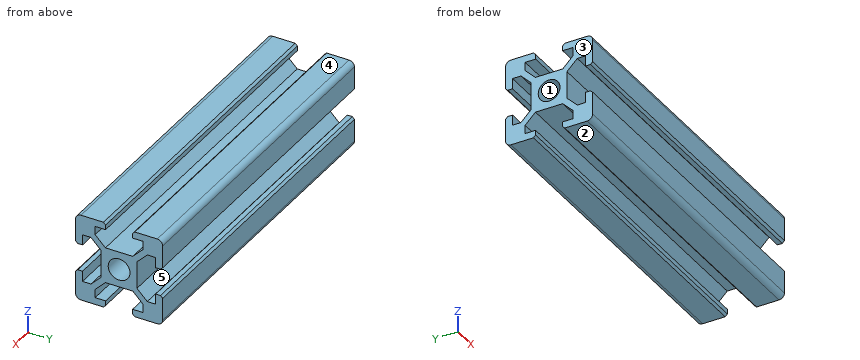
Autodesk Inventor part; units mm, degrees
ref_plane "YZ Plane" through (0, 0, 0) normal (1, 0, 0) x (0, 1, 0)
ref_plane "XZ Plane" through (0, 0, 0) normal (0, 1, 0) x (-1, 0, 0)
ref_plane "XY Plane" through (0, 0, 0) normal (0, 0, 1) x (1, 0, 0)
sketch "Sketch1" plane through (0, 0, 0) normal (1, 0, 0) x (0, 1, 0)
  circle A0 centre (0, 0) radius 2.5
  line L0 (0, 0) -> (10, 0)
  line L1 (10, -10) -> (10, -3.6)
  line L2 (10, -3.6) -> (9.5, -3.1)
  line L3 (9.5, -3.1) -> (8.4, -3.1)
  line L4 (8.4, -3.1) -> (8.4, -5.5)
  line L5 (-3.134, 4.1) -> (3.134, 4.1)
  line L6 (4.1, 3.134) -> (4.1, -3.134)
  line L7 (3.134, -4.1) -> (-3.134, -4.1)
  line L8 (-4.1, -3.134) -> (-4.1, 3.134)
  line L9 (-4.1, 4.1) -> (4.1, -4.1) construction
  line L10 (4.1, 4.1) -> (-4.1, -4.1) construction
  line L11 (4.1, -3.134) -> (6.466, -5.5)
  line L12 (8.4, -5.5) -> (6.466, -5.5)
  line L13 (10, -10) -> (3.6, -10)
  line L14 (3.6, -10) -> (3.1, -9.5)
  line L15 (3.1, -9.5) -> (3.1, -8.4)
  line L16 (3.1, -8.4) -> (5.5, -8.4)
  line L17 (3.134, -4.1) -> (5.5, -6.466)
  line L18 (5.5, -8.4) -> (5.5, -6.466)
  line L19 (10, 10) -> (10, 3.6)
  line L20 (10, 3.6) -> (9.5, 3.1)
  line L21 (9.5, 3.1) -> (8.4, 3.1)
  line L22 (8.4, 3.1) -> (8.4, 5.5)
  line L23 (4.1, 3.134) -> (6.466, 5.5)
  line L24 (8.4, 5.5) -> (6.466, 5.5)
  line L25 (5.5, 8.4) -> (5.5, 6.466)
  line L26 (3.134, 4.1) -> (5.5, 6.466)
  line L27 (3.1, 8.4) -> (5.5, 8.4)
  line L28 (3.1, 9.5) -> (3.1, 8.4)
  line L29 (3.6, 10) -> (3.1, 9.5)
  line L30 (10, 10) -> (3.6, 10)
  line L31 (0, 0) -> (0, -5.5)
  line L32 (-10, -10) -> (-10, -3.6)
  line L33 (-10, -3.6) -> (-9.5, -3.1)
  line L34 (-9.5, -3.1) -> (-8.4, -3.1)
  line L35 (-8.4, -3.1) -> (-8.4, -5.5)
  line L36 (-4.1, -3.134) -> (-6.466, -5.5)
  line L37 (-8.4, -5.5) -> (-6.466, -5.5)
  line L38 (-5.5, -8.4) -> (-5.5, -6.466)
  line L39 (-3.134, -4.1) -> (-5.5, -6.466)
  line L40 (-3.1, -8.4) -> (-5.5, -8.4)
  line L41 (-3.1, -9.5) -> (-3.1, -8.4)
  line L42 (-3.6, -10) -> (-3.1, -9.5)
  line L43 (-10, -10) -> (-3.6, -10)
  line L44 (-4.1, 3.134) -> (-6.466, 5.5)
  line L45 (-3.134, 4.1) -> (-5.5, 6.466)
  line L46 (-8.4, 3.1) -> (-8.4, 5.5)
  line L47 (-8.4, 5.5) -> (-6.466, 5.5)
  line L48 (-5.5, 8.4) -> (-5.5, 6.466)
  line L49 (-3.1, 8.4) -> (-5.5, 8.4)
  line L50 (-9.5, 3.1) -> (-8.4, 3.1)
  line L51 (-10, 3.6) -> (-9.5, 3.1)
  line L52 (-3.1, 9.5) -> (-3.1, 8.4)
  line L53 (-3.6, 10) -> (-3.1, 9.5)
  line L54 (-10, 10) -> (-3.6, 10)
  line L55 (-10, 10) -> (-10, 3.6)
  point P0 (-10, 0)
  dimension "d0" = 5
  dimension "d3" = 3.6
  dimension "d4" = 45
  dimension "d5" = 3.1
  dimension "d7" = 5.5
  dimension "d8" = 1.6
  dimension "d11" = 4.3
extrude "Extrusion1" add sketch "Sketch1" along normal blind 76.2 contours L0 L6 L11 L12 L4 L3 L2 L1 L13 L14 L15 L16 L18 L17 L7 L31 A0 | A0 L31 L7 L39 L38 L40 L41 L42 L43 L32 L33 L34 L35 L37 L36 L8 L44 L47 L46 L50 L51 L55 L54 L53 L52 L49 L48 L45 L5 L26 L25 L27 L28 L29 L30 L19 L20 L21 L22 L24 L23 L6 L0
fillet "Fillet1" radius 1.25 4 edges at (38.1, 10, 10) (38.1, -10, 10) (38.1, 10, -10) (38.1, -10, -10)
properties part number "2020-3in"
Input: part model. Units: mm. Frame: model coordinates. Face numbers are marked on the shaded views. A direction names the side the tool comes from. Round coordinates to 2 decimals unless told otherwise and drop trailing zeros. Write each loop counter-clockwise with the first axis right and the second up, starting at its lowest first coordinate (ties: lowest second). Pieces come first, ordered by that corner, then holes.
1) Contact query for flat-ended pins moving along their axis: P1, Ø8, axis at x = 55.5, z = 1.5, coming from the -Y side; P2, Ø1.5, axis at y = -7, z = 2.5, coming from the -X side; P3, Ø2, axis at x = 20, z = 0, coming from the +Y side; P4, Ø3, axis at x = 36, z = -0.5, coming from the -Y side. Output: stop coordinate, or through.
2) Cut plane B-B (y = 0). Return the cut outline in (x, z).
3) Cut plane A-A (z = -1.5). Return the cut outline in (x, y).
4) Draft query along Z for the marked faces 1, 2 and 3. Return one class per face: pulls with the +Z half, pulls with the -Z half, needs draft (parallel to the pull), parting line crosses it, or undercut.
5) Ray query, L1, parallel to Z at x = 33.5, y = 0; L2, parallel to Z at x = 44.5, y = -7. Return the intervals inside material, ascending.
6) Reachability of the marked faces 4 and 5 from +Z, -Z, +X, -X, +Y, -Y: full face, straight path, thin tool, end or side. Return the list, or none.
Geometry says:
1. P1: stops at y = -10
1. P2: passes through
1. P3: stops at y = 4.1
1. P4: stops at y = -4.1
2. outline: (0, -4.1) - (76.2, -4.1) - (76.2, -2.5) - (0, -2.5) - close; (0, 2.5) - (76.2, 2.5) - (76.2, 4.1) - (0, 4.1) - close
3. outline: (0, -4.1) - (76.2, -4.1) - (76.2, -2) - (0, -2) - close; (0, 2) - (76.2, 2) - (76.2, 4.1) - (0, 4.1) - close
4. face 1: undercut
4. face 2: pulls with the -Z half
4. face 3: needs draft
5. L1: z = -4.1 to -2.5, 2.5 to 4.1
5. L2: z = -10 to -5.5, 5.5 to 10
6. face 4: +Z, +X, -X, +Y, -Y
6. face 5: +X, -X
